The listing builds one solid part. Answer for the finished solid, in the listing's coordinates (mm). Round coordinates to 2 decimals unless told otherwise and drop trailing zeros. Write each loop counter-clockwise with the first axis right and the second up, starting at its lowest first coordinate (ties: lowest second). Pieces come first, ordered by that corner, then holes. Notation, with made-up numbers: (-24.75, -3.5) -> (2.25, -3.5) arc R24 ccw to (2.25, 27.5) -> close; hole circle Ø3 at (54, 41.5). An arc over 180 degrees is marked (long way). Write each question's results on one line, items separated by ' | '. Start each with the question number.
```python
from build123d import *

# Parameters (mm, degrees)
SKETCH1_W           = 24
SKETCH1_H           = 6
SKETCH1_W_2         = 23
SKETCH1_H_2         = 3
BOSS_EXTRUDE1_DEPTH = 3


with BuildPart() as part:
    # Sketch1 → Boss-Extrude1 (new body)
    with BuildSketch(Plane(origin=(0, 0, 0), x_dir=(1, 0, 0), z_dir=(0, 1, 0))):
        Polygon((-45.497230944, 18), (-66.994461887, 18), (-66.994461887, 0), (-45.497230944, 0), (-22.497230944, 0), (-21.497230944, 0), (0, 0), (0, 18), (-21.497230944, 18), align=None)
        with Locations((-33.497230944, 21)):
            Rectangle(SKETCH1_W, SKETCH1_H)
        with Locations((-33.997230944, -1.5)):
            Rectangle(SKETCH1_W_2, SKETCH1_H_2)
    extrude(amount=BOSS_EXTRUDE1_DEPTH)


solid = part.part
```
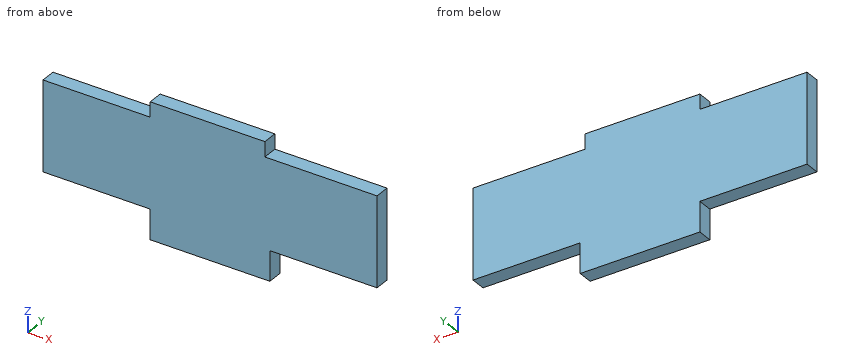
Q1. Each of these flat-tipped pins is pushed along its axis until it touches: pin 1 (0.9 mm diameter, centred on x = -56, y = 2, fed in from +Z); pin 2 (1.5 mm diameter, centred on y = 2, z = -22.5, fed in from -X). Where does it stop, or does it pass through?
Q2. The part is cut by section B-B, the plane z = -20.75. Write down the section's boundary in (x, y), then the cut area to 3 significant figures.
Q3. The part is cut by section C-C, the plane x = -59.5. Write down the section's boundary in (y, z), then the cut area to 3 significant figures.
Q4. The part is cut by section A-A, the plane y = 1.2. Write down the section's boundary in (x, z), then the cut area to 3 significant figures.
Q5. Find the intervals of material crossed by line 1 (Z direction, x = -59.5, y = 0.85); line 2 (X direction, y = 0.9, z = -18.5); line 3 (Z direction, x = -22, y = 1.65), in increasing order.
Answers follow:
1) pin 1: z = 0 | pin 2: x = -45.5
2) outline: (-45.5, 0) -> (-21.5, 0) -> (-21.5, 3) -> (-45.5, 3) -> close | area: 72.0 mm^2
3) outline: (0, -18) -> (3, -18) -> (3, 0) -> (0, 0) -> close | area: 54.0 mm^2
4) outline: (-66.99, -18) -> (-45.5, -18) -> (-45.5, -24) -> (-21.5, -24) -> (-21.5, -18) -> (0, -18) -> (0, 0) -> (-22.5, 0) -> (-22.5, 3) -> (-45.5, 3) -> (-45.5, 0) -> (-66.99, 0) -> close | area: 1,420 mm^2
5) line 1: -18 to 0 | line 2: -45.5 to -21.5 | line 3: -24 to 0
